from build123d import *

# Parameters (mm, degrees)
SKETCH_1_W          = 50
SKETCH_1_H          = 50
SKETCH_1_R          = 21.05
EXTRUDE_1_DEPTH     = 5
SKETCH_2_W          = 50
SKETCH_2_H          = 30
SKETCH_2_R          = 1.45
EXTRUDE_2_DEPTH     = 5
FILLET_1_R          = 3
EXTRUDE_START       = -5
SKETCH_4_R          = 21.05
EXTRUDE_3_DEPTH     = 5
SKETCH_5_R          = 13.25
SKETCH_5_R_2        = 2.1
CUT_EXTRUDE_2_DEPTH = 61.621778265
SKETCH_6_R          = 1.45
CUT_EXTRUDE_3_DEPTH = 61.621778265
CUT_EXTRUDE_4_DEPTH = 61.621778265
SKETCH_8_W          = 6
SKETCH_8_H          = 17.5
EXTRUDE_4_DEPTH     = 5
FILLET_2_R          = 2


with BuildPart() as part:
    # 草图1 → 凸台-拉伸1 (new body)
    with BuildSketch(Plane(origin=(0, 0, 0), x_dir=(1, 0, 0), z_dir=(0, 1, 0))):
        Rectangle(SKETCH_1_W, SKETCH_1_H)
        with Locations(Location((0, 0, 0), (0, 0, 270))):
            Circle(SKETCH_1_R, mode=Mode.SUBTRACT)
    extrude(amount=EXTRUDE_1_DEPTH)

    # 草图2 → 凸台-拉伸2 (add)
    with BuildSketch(Plane(origin=(0, 5, 0), x_dir=(1, 0, 0), z_dir=(0, 1, 0))):
        with Locations((0, -40)):
            Rectangle(SKETCH_2_W, SKETCH_2_H)
        with Locations(Location((-15, -47.5, 0), (0, 0, 270))):
            Circle(SKETCH_2_R, mode=Mode.SUBTRACT)
        with Locations(Location((15, -47.5, 0), (0, 0, 270))):
            Circle(SKETCH_2_R, mode=Mode.SUBTRACT)
    extrude(amount=-EXTRUDE_2_DEPTH)

    # 圆角1
    fillet_1_edges = [part.edges().sort_by_distance(p)[0] for p in [
        (25, 2.5, 55),
        (-25, 2.5, 55),
        (-25, 2.5, -25),
        (25, 2.5, -25),
    ]]
    fillet(fillet_1_edges, radius=FILLET_1_R)

    # 草图4 → 凸台-拉伸3 (add)
    with BuildSketch(Plane(origin=(0, 5, 0), x_dir=(1, 0, 0), z_dir=(0, 1, 0)).offset(EXTRUDE_START)):
        Circle(SKETCH_4_R)
    extrude(amount=EXTRUDE_3_DEPTH)

    # 草图5 → 切除-拉伸2 (cut, through all)
    with BuildSketch(Plane.XZ):
        with Locations(Location((0, 0, 0), (0, 0, 270))):
            Circle(SKETCH_5_R)
        with Locations(Location((0, 17.5, 0), (0, 0, 270))):
            Circle(SKETCH_5_R_2)
        with Locations(Location((17.5, 0, 0), (0, 0, 270))):
            Circle(SKETCH_5_R_2)
        with Locations(Location((0, -17.5, 0), (0, 0, 270))):
            Circle(SKETCH_5_R_2)
        with Locations(Location((-17.5, 0, 0), (0, 0, 270))):
            Circle(SKETCH_5_R_2)
    extrude(amount=-CUT_EXTRUDE_2_DEPTH, mode=Mode.SUBTRACT)

    # 草图6 → 切除-拉伸3 (cut, through all)
    with BuildSketch(Plane(origin=(0, 5, 0), x_dir=(1, 0, 0), z_dir=(0, 1, 0))):
        with Locations(Location((-15, -30, 0), (0, 0, 270))):
            Circle(SKETCH_6_R)
        with Locations(Location((15, -30, 0), (0, 0, 270))):
            Circle(SKETCH_6_R)
    extrude(amount=-CUT_EXTRUDE_3_DEPTH, mode=Mode.SUBTRACT)

    # 草图7 → 切除-拉伸4 (cut, through all)
    with BuildSketch(Plane(origin=(0, 5, 0), x_dir=(1, 0, 0), z_dir=(0, 1, 0))):
        with BuildLine():
            Line((8.55, -30), (-8.55, -30))
            ThreePointArc((-8.55, -30), (-10.439161261, -34.560838739), (-15, -36.45))
            Line((-15, -36.45), (-15, -41.05))
            ThreePointArc((-15, -41.05), (-10.439161261, -42.939161261), (-8.55, -47.5))
            Line((-8.55, -47.5), (8.55, -47.5))
            ThreePointArc((8.55, -47.5), (10.439161261, -42.939161261), (15, -41.05))
            Line((15, -41.05), (15, -36.45))
            ThreePointArc((15, -36.45), (10.439161261, -34.560838739), (8.55, -30))
        make_face()
    extrude(amount=-CUT_EXTRUDE_4_DEPTH, mode=Mode.SUBTRACT)

    # 草图8 → 凸台-拉伸4 (add)
    with BuildSketch(Plane(origin=(0, 5, 0), x_dir=(1, 0, 0), z_dir=(0, 1, 0))):
        with Locations((0, -38.75)):
            Rectangle(SKETCH_8_W, SKETCH_8_H)
    extrude(amount=-EXTRUDE_4_DEPTH)

    # 圆角2
    fillet_2_edges = [part.edges().sort_by_distance(p)[0] for p in [
        (-8.55, 2.5, 47.5),
        (-15, 2.5, 41.05),
        (-15, 2.5, 36.45),
        (-8.55, 2.5, 30),
        (8.55, 2.5, 30),
        (15, 2.5, 36.45),
        (15, 2.5, 41.05),
        (8.55, 2.5, 47.5),
        (-3, 2.5, 30),
        (3, 2.5, 30),
        (3, 2.5, 47.5),
        (-3, 2.5, 47.5),
    ]]
    fillet(fillet_2_edges, radius=FILLET_2_R)


solid = part.part
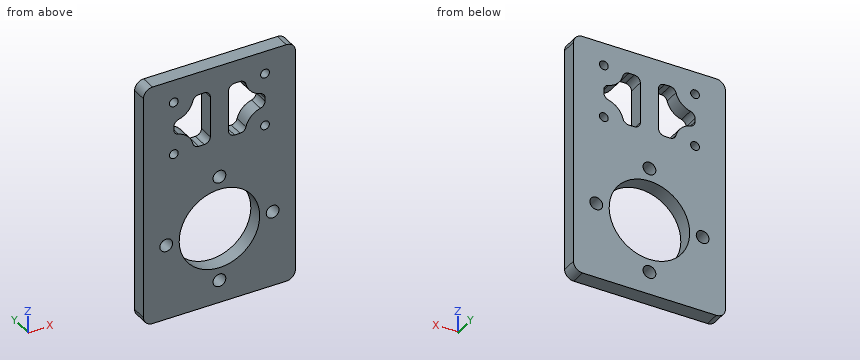
Geometry: final body of the model. Coordinates: model frame, mm. Round coordinates to 2 decimals unless told otherwise and drop trailing zeros. Loops run counter-clockwise (first coordinate to the right, second up) from the corner with the lowest first, then second, coordinate; pieces in that order, holes last.
Q1. Section B-B on x = -17.5. Return loops of the section in (y, z).
Q2. Section A-A on z = 17.5. Return loops of the section in (x, y).
Q3. Pin query (flat end, axial travel): P1, Ø2.5, axis at x = -15, z = 47.5, coming from the +Y side; P2, Ø4, axis at x = 15, z = 47.5, coming from the +Y side. Return the tip coordinate at first contact, or that it passes through.
Q4. Material intervals for L1, parallel to X at y = 2.45, z = 0; L2, parallel to X at y = 2.6, z = -17.5; L3, parallel to X at y = 1.7, z = 41, sorted ascending.
Q5. Section C-C on x = 0. Return loops of the section in (y, z).
Q6. Section D-D on y = 0.8. State how many separate pieces and enclosed holes the cut face has, plus the area to 3 significant figures.
Evaluation:
1. outline: (0, -25) - (5, -25) - (5, -2.1) - (0, -2.1) - close; (0, 2.1) - (5, 2.1) - (5, 55) - (0, 55) - close
2. outline: (-25, 0) - (-2.1, 0) - (-2.1, 5) - (-25, 5) - close; (2.1, 0) - (25, 0) - (25, 5) - (2.1, 5) - close
3. P1: passes through
3. P2: stops at y = 5
4. L1: x = -25 to -19.6, -15.4 to -13.25, 13.25 to 15.4, 19.6 to 25
4. L2: x = -25 to -2.1, 2.1 to 25
4. L3: x = -25 to -14.04, -3 to 3, 14.04 to 25
5. outline: (0, -25) - (5, -25) - (5, -19.6) - (0, -19.6) - close; (0, -15.4) - (5, -15.4) - (5, -13.25) - (0, -13.25) - close; (0, 13.25) - (5, 13.25) - (5, 15.4) - (0, 15.4) - close; (0, 19.6) - (5, 19.6) - (5, 55) - (0, 55) - close
6. separate pieces: 1
6. enclosed holes: 11
6. area: 3,080 mm2
